Geometry check sheet. Reference: the model listing, model coordinates, mm. Round coordinates to 2 decimals unless told otherwise and drop trailing zeros. Loops run counter-clockwise (first coordinate to the right, second up) from the corner with the lowest first, then second, coordinate; pieces in that order, holes last. Notation, with made-up numbers: (5, 62.5) -> (22, 62.5) arc R22 cw to (22, 73.5) -> close; hole circle Ø1 at (69, 75). An arc over 180 degrees is marked (long way). Use a Markdown table: item, result. Add a question column.
Q1. Sectioned sample at C-C, the plane z = 0.25. Enter the section's corners in (x, y) (3 decimals), then the cut area to 3 significant figures.
Q2. Sectioned sample at A-A, the plane x = 0. Enter the section's corners in (y, z), then the cut area to 4 significant figures.
Q3. Material ranges on L1, parallel to X at y = -0.75, z = -5 (3 decimals); L2, parallel to X at y = 1.5, z = 0.5 (3 decimals); L3, parallel to Y at x = 0, z = -1.5, recorded low to high.
Q4. Sectioned sample at B-B, the plane y = 0. Enter the section's corners in (x, z) (3 decimals), then the cut area to 3 significant figures.
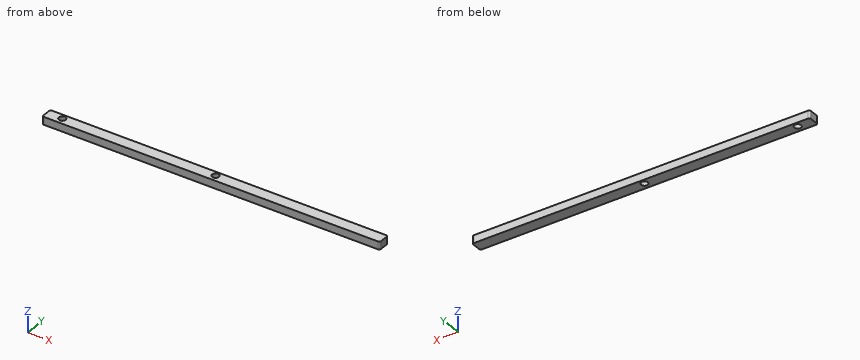
```python
from build123d import *

# Parameters (mm, degrees)
SKETCH1_W           = 552.45
SKETCH1_H           = 19.05
SKETCH1_R           = 5.588
BOSS_EXTRUDE1_DEPTH = 6.35
FILLET1_R           = 2.54


with BuildPart() as part:
    # Sketch1 → Boss-Extrude1 (new, symmetric)
    with BuildSketch(Plane.XY):
        with Locations((0, -1.257859134)):
            Rectangle(SKETCH1_W, SKETCH1_H)
        Circle(SKETCH1_R, mode=Mode.SUBTRACT)
        with Locations((-250.825, 0)):
            Circle(SKETCH1_R, mode=Mode.SUBTRACT)
    extrude(amount=BOSS_EXTRUDE1_DEPTH, both=True)

    # Fillet1
    fillet1_edges = [part.edges().sort_by_distance(p)[0] for p in [
        (276.225, -10.782859134, 0),
        (-276.225, -10.782859134, 0),
        (-276.225, 8.267140866, 0),
        (276.225, 8.267140866, 0),
    ]]
    fillet(fillet1_edges, radius=FILLET1_R)


solid = part.part
```
Values:
| question | item | result |
|---|---|---|
| 1 | outline | (-276.225, -8.243) arc R2.54 ccw to (-273.685, -10.783) -> (273.685, -10.783) arc R2.54 ccw to (276.225, -8.243) -> (276.225, 5.727) arc R2.54 ccw to (273.685, 8.267) -> (-273.685, 8.267) arc R2.54 ccw to (-276.225, 5.727) -> close; hole circle Ø11.176 at (-250.825, 0); hole circle Ø11.176 at (0, 0) |
| 1 | area | 10,300 mm^2 |
| 2 | outline | (-10.78, -6.35) -> (-5.59, -6.35) -> (-5.59, 6.35) -> (-10.78, 6.35) -> close; (5.59, -6.35) -> (8.27, -6.35) -> (8.27, 6.35) -> (5.59, 6.35) -> close |
| 2 | area | 100.0 mm^2 |
| 3 | L1 | -276.225 to -256.362, -245.288 to -5.537, 5.537 to 276.225 |
| 3 | L2 | -276.225 to -256.208, -245.442 to -5.383, 5.383 to 276.225 |
| 3 | L3 | -10.78 to -5.59, 5.59 to 8.27 |
| 4 | outline | (-276.225, -6.35) -> (-256.413, -6.35) -> (-256.413, 6.35) -> (-276.225, 6.35) -> close; (-245.237, -6.35) -> (-5.588, -6.35) -> (-5.588, 6.35) -> (-245.237, 6.35) -> close; (5.588, -6.35) -> (276.225, -6.35) -> (276.225, 6.35) -> (5.588, 6.35) -> close |
| 4 | area | 6,730 mm^2 |
